Geometry check sheet. Reference: the model listing, model coordinates, mm. A direction names the side the tool comes from. Give positions to 0.01 mm unless a question says otherwise; leave off trailing zeros. Write each loop counter-clockwise with the first axis right and the second up, starting at its lowest first coordinate (ties: lowest second). Pieces come first, ordered by that corner, then holes. Notation, with made-up numbers: (-1, 32.5) - (22, 32.5) arc R28 cw to (22, 63.5) - close; hole circle Ø5 at (80.5, -9.75). An arc over 180 degrees is marked (long way). Use a Markdown table: item, result.
```python
from build123d import *

# Parameters (mm, degrees)
SKETCH1_R             = 18.5
SKETCH1_R_2           = 5
BOSS_EXTRUDE1_DEPTH   = 3
SKETCH1_R_3           = 20.5
BOSS_EXTRUDE1_2_DEPTH = 3
BOSS_EXTRUDE2_DEPTH   = 3


with BuildPart() as part:
    # Sketch1 → Boss-Extrude1 (new body)
    with BuildSketch(Plane(origin=(0, 0, 0), x_dir=(1, 0, 0), z_dir=(0, 1, 0))):
        with Locations((20.568259386, 26.155290102)):
            Circle(SKETCH1_R)
        with Locations((20.568259386, 26.155290102)):
            Circle(SKETCH1_R_2, mode=Mode.SUBTRACT)
    extrude(amount=BOSS_EXTRUDE1_DEPTH)



with BuildPart() as body_2:
    # Sketch1 → Boss-Extrude1 2 (new body)
    with BuildSketch(Plane(origin=(0, 0, 0), x_dir=(1, 0, 0), z_dir=(0, 1, 0))):
        Polygon((-16.931740614, 39.155290102), (-1.931740614, 54.155290102), (43.068259386, 54.155290102), (58.068259386, 39.155290102), (58.068259386, -0.844709898), (-16.931740614, -0.844709898), align=None)
        with Locations((20.568259386, 26.155290102)):
            Circle(SKETCH1_R_3, mode=Mode.SUBTRACT)
    extrude(amount=BOSS_EXTRUDE1_2_DEPTH)


with BuildPart() as part_1:
    add(part.part)

    add(body_2.part)  # Boss-Extrude2 merges body 2
    # Sketch2 → Boss-Extrude2 (add, through all)
    with BuildSketch(Plane(origin=(0, 3, 0), x_dir=(1, 0, 0), z_dir=(0, 1, 0))):
        with BuildLine():
            Line((18.068259386, 44.485592882), (18.068259386, 46.502280052))
            ThreePointArc((18.068259386, 46.502280052), (20.568259386, 46.655290102), (23.068259386, 46.502280052))
            Line((23.068259386, 46.502280052), (23.068259386, 44.485592882))
            ThreePointArc((23.068259386, 44.485592882), (20.568259386, 44.655290102), (18.068259386, 44.485592882))
        make_face()
        with BuildLine():
            Line((35.192767252, 37.485505002), (36.939269572, 38.493848587))
            ThreePointArc((36.939269572, 38.493848587), (38.321780163, 36.405290102), (39.439269572, 34.163721568))
            Line((39.439269572, 34.163721568), (37.692767252, 33.155377983))
            ThreePointArc((37.692767252, 33.155377983), (36.589729356, 35.405290102), (35.192767252, 37.485505002))
        make_face()
        with BuildLine():
            Line((37.692767252, 19.155202222), (39.439269572, 18.146858637))
            ThreePointArc((39.439269572, 18.146858637), (38.321780163, 15.905290102), (36.939269572, 13.816731618))
            Line((36.939269572, 13.816731618), (35.192767252, 14.825075203))
            ThreePointArc((35.192767252, 14.825075203), (36.589729356, 16.905290102), (37.692767252, 19.155202222))
        make_face()
        with BuildLine():
            Line((23.068259386, 7.824987323), (23.068259386, 5.808300153))
            ThreePointArc((23.068259386, 5.808300153), (20.568259386, 5.655290102), (18.068259386, 5.808300153))
            Line((18.068259386, 5.808300153), (18.068259386, 7.824987323))
            ThreePointArc((18.068259386, 7.824987323), (20.568259386, 7.655290102), (23.068259386, 7.824987323))
        make_face()
        with BuildLine():
            Line((5.943751519, 14.825075203), (4.197249199, 13.816731618))
            ThreePointArc((4.197249199, 13.816731618), (2.814738608, 15.905290102), (1.697249199, 18.146858637))
            Line((1.697249199, 18.146858637), (3.443751519, 19.155202222))
            ThreePointArc((3.443751519, 19.155202222), (4.546789416, 16.905290102), (5.943751519, 14.825075203))
        make_face()
        with BuildLine():
            Line((3.443751519, 33.155377983), (1.697249199, 34.163721568))
            ThreePointArc((1.697249199, 34.163721568), (2.814738608, 36.405290102), (4.197249199, 38.493848587))
            Line((4.197249199, 38.493848587), (5.943751519, 37.485505002))
            ThreePointArc((5.943751519, 37.485505002), (4.546789416, 35.405290102), (3.443751519, 33.155377983))
        make_face()
    extrude(amount=-BOSS_EXTRUDE2_DEPTH)


solid = part_1.part
```
1) Material ranges on L1, parallel to X at y = 0.7, z = -26; L2, parallel to Z at x = 28, y = 1.55; L3, parallel to X at y = 2.85, z = -28.5, recorded low to high. Write a range as from..to.
Working result:
| item | result |
|---|---|
| L1 | x = -16.93..0.07, 2.07..15.57, 25.57..39.07, 41.07..58.07 |
| L2 | z = -54.16..-45.26, -43.1..-9.21, -7.05..0.84 |
| L3 | x = -16.93..0.2, 2.22..16.15, 24.98..38.92, 40.93..58.07 |
2) Section check D-D on z = -12.5. Record the boundary of the cut face in (x, y).
Working result:
| item | result |
|---|---|
| outline | (-16.93, 0) - (5.28, 0) - (5.28, 3) - (-16.93, 3) - close; (8.09, 0) - (33.05, 0) - (33.05, 3) - (8.09, 3) - close; (35.86, 0) - (58.07, 0) - (58.07, 3) - (35.86, 3) - close |
3) Set-up check for faces 4 (the flat face through (21, 0, -21)), 5 (the cylindrical face through (10.418, 1.479, -43.966)): record each of +Z, -Z, +X, -X, +Y, -Y from which the full face is reachable in a straight line by a thin tool's end or side.
Working result:
| item | result |
|---|---|
| face 4 | +Z, -Z, +X, -X, -Y |
| face 5 | +Y, -Y |
4) Mould release check, pull along X, two halves, no side actions. Record for faces 1 (the flat face through (58.068, 1, -19)), 2 (the flat face through (36.05, 1.52, -37.98)), 3 (the flat face through (-9.537, 1.479, -46.55)): pulls with the +X half, pulls with the -X half, needs draft (parallel to the pull), parting line crosses it, or undercut.
Working result:
| item | result |
|---|---|
| face 1 | pulls with the +X half |
| face 2 | undercut |
| face 3 | pulls with the -X half |
5) Section check A-A on z = -24. Record the boundary of the cut face in (x, y), then the cut area to 3 significant figures.
Working result:
| item | result |
|---|---|
| outline | (-16.93, 0) - (0.18, 0) - (0.18, 3) - (-16.93, 3) - close; (2.19, 0) - (16.06, 0) - (16.06, 3) - (2.19, 3) - close; (25.08, 0) - (38.94, 0) - (38.94, 3) - (25.08, 3) - close; (40.95, 0) - (58.07, 0) - (58.07, 3) - (40.95, 3) - close |
| area | 186 mm² |
6) Depth check by flat-ended pin: P1, Ø0.6, axis at y = 1.5, z = -46, coming from the -X side. Enter the tip coordinate at first touch or a pass-through.
Working result:
| item | result |
|---|---|
| P1 | stops at x = -10.39 |
7) Section check B-B on x = 8.5. Record the boundary of the cut face in (y, z).
Working result:
| item | result |
|---|---|
| outline | (0, -54.16) - (3, -54.16) - (3, -42.73) - (0, -42.73) - close; (0, -40.18) - (3, -40.18) - (3, -12.13) - (0, -12.13) - close; (0, -9.58) - (3, -9.58) - (3, 0.84) - (0, 0.84) - close |
8) Section check C-C on y = 0.7. Count the separate pieces of the cut face and the enclosed holes in it, then the cut area to 3 significant figures.
Working result:
| item | result |
|---|---|
| separate pieces | 1 |
| enclosed holes | 7 |
| area | 3,640 mm² |
